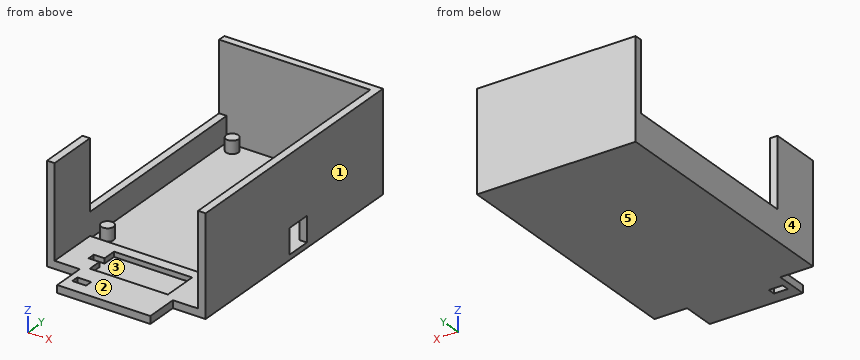
```python
from build123d import *

# Parameters (mm, degrees)
P_IDAT_VYSUNUT_M1_DEPTH  = 2
SKICA3_R                 = 2.45
P_IDAT_VYSUNUT_M3_DEPTH  = 5
P_IDAT_VYSUNUT_M4_DEPTH  = 37.5
SKICA8_W                 = 10
SKICA8_H                 = 10
ODEBRAT_VYSUNUT_M2_DEPTH = 136.974087605
SKICA10_W                = 27.5
SKICA10_H                = 79
ODEBRAT_VYSUNUT_M3_DEPTH = 3
P_IDAT_VYSUNUT_M5_DEPTH  = 1
ODEBRAT_VYSUNUT_M4_DEPTH = 2
SKICA12_3_W              = 5.5
SKICA12_3_H              = 3
ODEBRAT_VYSUNUT_M5_DEPTH = 137.49158399


with BuildPart() as part:
    # Skica1 → Přidat vysunutím1 (new body)
    with BuildSketch(Plane.XY):
        Polygon((13, -102.45), (13, -115.45), (50, -115.45), (50, -102.45), (63, -102.45), (63, 0), (0, 0), (0, -102.45), align=None)
    extrude(amount=P_IDAT_VYSUNUT_M1_DEPTH)

    # Skica3 → Přidat vysunutím3 (add)
    with BuildSketch(Plane.XY.offset(2)):
        with Locations((7.55, -6.45)):
            Circle(SKICA3_R)
        with Locations((7.55, -78.45)):
            Circle(SKICA3_R)
        with Locations((55.55, -78.45)):
            Circle(SKICA3_R)
        with Locations((55.55, -6.45)):
            Circle(SKICA3_R)
    extrude(amount=P_IDAT_VYSUNUT_M3_DEPTH)

    # Skica4 → Přidat vysunutím4 (add)
    with BuildSketch(Plane.XY.offset(2)):
        Polygon((63, 0), (63, -102.45), (60, -102.45), (60, -3), (3, -3), (3, -102.45), (0, -102.45), (0, 0), align=None)
    extrude(amount=P_IDAT_VYSUNUT_M4_DEPTH)

    # Skica8 → Odebrat vysunutím2 (cut, through all)
    with BuildSketch(Plane.ZY.offset(-60)):
        with Locations((7, -49)):
            Rectangle(SKICA8_W, SKICA8_H)
    extrude(amount=-ODEBRAT_VYSUNUT_M2_DEPTH, mode=Mode.SUBTRACT)

    # Skica10 → Odebrat vysunutím3 (cut)
    with BuildSketch(Plane.ZY):
        with Locations((25.75, -42.5)):
            Rectangle(SKICA10_W, SKICA10_H)
    extrude(amount=-ODEBRAT_VYSUNUT_M3_DEPTH, mode=Mode.SUBTRACT)

    # Skica11 → Přidat vysunutím5 (add)
    with BuildSketch(Plane.XY.offset(2)):
        Polygon((3, -82), (60, -82), (60, -102.45), (50, -102.45), (50, -115.45), (13, -115.45), (13, -102.45), (3, -102.45), align=None)
    extrude(amount=P_IDAT_VYSUNUT_M5_DEPTH)

    # Skica12 → Odebrat vysunutím4 (cut)
    with BuildSketch(Plane.XY.offset(3)):
        Polygon((15.5, -86.25), (15.5, -91.75), (11.2, -91.75), (11.2, -94.75), (15.5, -94.75), (15.5, -100.25), (46.5, -100.25), (46.5, -86.25), align=None)
    extrude(amount=-ODEBRAT_VYSUNUT_M4_DEPTH, mode=Mode.SUBTRACT)

    # Skica12<3> → Odebrat vysunutím5 (cut, through all)
    with BuildSketch(Plane.XY.offset(3)):
        with Locations((18.25, -108.95)):
            Rectangle(SKICA12_3_W, SKICA12_3_H)
    extrude(amount=-ODEBRAT_VYSUNUT_M5_DEPTH, mode=Mode.SUBTRACT)


solid = part.part
```
CAD build for the part. Positions are in the model's coordinates, mm. Face numbers are marked on the shaded views. A direction names the side the tool comes from. Coordinates: 2 decimals unless noted, no trailing zeros. Loops run counter-clockwise (first coordinate to the right, second up) from the corner with the lowest first, then second, coordinate; pieces in that order, holes last. Notation, with made-up numbers: (20, 87) - (47, 87) arc R33 cw to (47, 119) - close; hole circle Ø1 at (-15, 67.25). An arc over 180 degrees is marked (long way). Return JSON: item names as keys, results as strings.
1. Mould opens along X. For the marked faces 3, 4 and 5 say: released by +X, released by -X, zero draft, split by the parting line, or undercut.
Result:
{"face 3": "undercut", "face 4": "released by -X", "face 5": "zero draft"}
2. Band-saw the part on C-C (x = 41). Give the cut face in (y, z), and give its area (3 significant figures).
Result:
{"outline": "(-115.45, 0) - (0, 0) - (0, 39.5) - (-3, 39.5) - (-3, 2) - (-82, 2) - (-82, 3) - (-86.25, 3) - (-86.25, 1) - (-100.25, 1) - (-100.25, 3) - (-115.45, 3) - close", "area": "349 mm2"}
3. 3-axis set-ups, long thin cutter, end or side, ignore diameter. For the marked faces 1 and 2: which of +Z, -Z, +X, -X, +Y, -Y reach the whole face in a straight line?
Result:
{"face 1": "+Z, -Z, +X, +Y, -Y", "face 2": "+Z, -Y"}
4. Probe L1, parallel to Y at x = 39, z = 29.5; L2, parallel to X at y = -101.5, z = 15; L3, parallel to Z at x = 55, y = -93. List the from-to ranges inside material, lowest first. Write a range as from..to.
Result:
{"L1": "y = -3..0", "L2": "x = 0..3, 60..63", "L3": "z = 0..3"}
5. Band-saw the part on A-A (z = 25). Give the cut face in (x, y).
Result:
{"outline": "(0, -102.45) - (3, -102.45) - (3, -82) - (0, -82) - close; (0, -3) - (60, -3) - (60, -102.45) - (63, -102.45) - (63, 0) - (0, 0) - close"}
6. Band-saw the part on B-B (y = -50.5). Give the cut face in (x, z), and give its area (4 significant figures).
Result:
{"outline": "(0, 0) - (63, 0) - (63, 2) - (3, 2) - (3, 12) - (0, 12) - close; (60, 12) - (63, 12) - (63, 39.5) - (60, 39.5) - close", "area": "238.5 mm2"}
7. Drop flat-ended pins along their axis: pin 1 (5 mm diameter, centred on x = 41, z = 16, fed in from +Y); pin 2 (4 mm diameter, centred on y = -23, z = 20, fed in from -X); pin 3 (2 mm diameter, centred on x = 48.5, z = 26, fed in from -Y); pin 4 (6.5 mm diameter, centred on x = 58.5, z = 29.5, fed in from -Y). Give the stop position or say it passes through.
Result:
{"pin 1": "stops at y = 0", "pin 2": "stops at x = 60", "pin 3": "stops at y = -3", "pin 4": "stops at y = -102.45"}
8. Band-saw the part on D-D (y = -6.45). Give the cut face in (x, z), and give its area (4 significant figures).
Result:
{"outline": "(0, 0) - (63, 0) - (63, 39.5) - (60, 39.5) - (60, 2) - (58, 2) - (58, 7) - (53.1, 7) - (53.1, 2) - (10, 2) - (10, 7) - (5.1, 7) - (5.1, 2) - (3, 2) - (3, 12) - (0, 12) - close", "area": "317.5 mm2"}
